```python
from build123d import *

# Parameters (mm, degrees)
F0_W     = 31.75
F0_H     = 31.75
F1_DEPTH = 57.15
F3_DEPTH = 12.7
F5_DEPTH = 12.7
F7_DEPTH = 12.7
F9_DEPTH = 12.7


with BuildPart() as f1:
    # F0 (on Front) → F1 (new body)
    with BuildSketch(Plane.XZ):
        with Locations((15.875, 15.875)):
            Rectangle(F0_W, F0_H)
    extrude(amount=F1_DEPTH)

    # F2 (on face) → F3 (cut)
    with BuildSketch(Plane(origin=(0, 0, 0), x_dir=(0, -1, 0), z_dir=(-1, 0, 0))):
        Polygon((57.15, 31.75), (19.05, 31.75), (31.75, 0), (57.15, 0), align=None)
    extrude(amount=-F3_DEPTH, mode=Mode.SUBTRACT)

    # F4 (on face) → F5 (cut)
    with BuildSketch(Plane.YZ.offset(19.05)):
        Polygon((-57.15, 0), (-19.05, 31.75), (-57.15, 31.75), align=None)
    extrude(amount=-F5_DEPTH, mode=Mode.SUBTRACT)

    # F6 (on face) → F7 (cut)
    with BuildSketch(Plane.YZ.offset(31.75)):
        Polygon((-57.15, 31.75), (-57.15, 0), (-19.05, 31.75), align=None)
    extrude(amount=-F7_DEPTH, mode=Mode.SUBTRACT)

    # F8 (on face) → F9 (cut)
    with BuildSketch(Plane.YZ.offset(31.75)):
        Polygon((-31.75, 0), (-19.05, 31.75), (-57.15, 0), align=None)
    extrude(amount=-F9_DEPTH, mode=Mode.SUBTRACT)


solid = f1.part
```
Input: part model. Units: mm. Frame: model coordinates. A direction names the side the tool comes from. Coordinates: 2 decimals unless noted, no trailing zeros. Loops run counter-clockwise (first coordinate to the right, second up) from the corner with the lowest first, then second, coordinate; pieces in that order, holes last. Notation, with made-up numbers: M 32.5,27 L 39.5,27 A19 ccw 39.5,59 Z; hole C 46.25,19.5 d3. An arc over 180 degrees is marked long. Use a Markdown table: item, result. Add a question column.
1) Section D-D, the plane y = -44.5. Return the cut outline in (x, z), plus the area to 3 significant figures.
2) Section C-C, the plane x = 16. Return the cut outline in (y, z), plus the area to 3 significant figures.
3) Set-up query: faces 1 (the flat face through (0, -12, 16)), 2 (the flat face through (25.49, -25.49, 15.65)), 3 (the flat face through (6.26, -25.31, 16.1)). Return all of +Z, -Z, +X, -X, +Y, -Y with unobstructed straight access to the full face (end or side cutting, diameter ignored); none if empty.
4) Section B-B, the plane z = 30. Return the cut outline in (x, y).
5) Section A-A, the plane z = 9.5. Return the cut outline in (x, y).
6) Line query: L1, parallel to X at y = -37, z = 6.5; L2, parallel to Y at x = 26.5, z = 22.5; L3, parallel to Y at x = 5.5, z = 9.5. Output: solid intervals per line, ascending. Write a range as from..to.
7) Pin query (flat end, axial travel): P1, Ø8, axis at y = -35, z = 26, coming from the -X side; P2, Ø9.5, axis at y = -35, z = 18.5, coming from the +X side; P3, Ø8, axis at x = 12.5, y = -25.5, coming from the +Z side; P4, Ø6, axis at x = 20, y = -50, coming from the +Z side. Return the tip coordinate at first contact, or that it passes through.
Answer below:
| question | item | result |
|---|---|---|
| 1 | outline | M 12.7,0 L 19.05,0 L 19.05,10.54 L 12.7,10.54 Z |
| 1 | area | 66.9 mm2 |
| 2 | outline | M -57.15,0 L 0,0 L 0,31.75 L -19.05,31.75 Z |
| 2 | area | 1,210 mm2 |
| 3 | face 1 | +Z, -Z, -X, +Y, -Y |
| 3 | face 2 | +Z, +X, -Y |
| 3 | face 3 | +Z, -X, -Y |
| 4 | outline | M 0,-19.75 L 12.7,-19.75 L 12.7,-21.15 L 19.05,-21.15 L 19.05,-19.75 L 31.75,-19.75 L 31.75,0 L 0,0 Z |
| 5 | outline | M 0,-27.95 L 12.7,-27.95 L 12.7,-45.75 L 19.05,-45.75 L 19.05,-27.95 L 31.75,-27.95 L 31.75,0 L 0,0 Z |
| 6 | L1 | 12.7..19.05 |
| 6 | L2 | -22.75..0 |
| 6 | L3 | -27.95..0 |
| 7 | P1 | through |
| 7 | P2 | x = 19.05 |
| 7 | P3 | z = 29.7 |
| 7 | P4 | z = 8.33 |
